Read the model definition and answer for the solid it produces. Units are mm, in the model's axes. Face numbers are marked on the shaded views. A direction names the side the tool comes from. Round coordinates to 2 decimals unless told otherwise and drop trailing zeros. Write each loop counter-clockwise with the first axis right and the second up, starting at its lowest first coordinate (ties: lowest second). Pieces come first, ordered by that corner, then holes. Notation, with made-up numbers: (83, -25) -> (132, -25) arc R34 cw to (132, 9) -> close; hole circle Ø3 at (40, 42). An arc over 180 degrees is marked (long way). Return JSON: item names as keys, results as strings.
from build123d import *

# Parameters (mm, degrees)
SKETCH1_R           = 49.53
BOSS_EXTRUDE1_DEPTH = 15.24
HEX_HOLE_DEPTH      = 13.97
SKETCH5_R           = 4.191
CENTERHOLE_DEPTH    = 72.425504548
SKETCH6_R           = 39.37
CUT_EXTRUDE1_DEPTH  = 11.43
SKETCH7_R           = 3.302
CUT_EXTRUDE2_DEPTH  = 72.684722222
SKETCH8_R           = 49.53
SKETCH8_R_2         = 39.37
CUT_EXTRUDE3_DEPTH  = 11.43
SKETCH9_R           = 49.53
SKETCH9_R_2         = 24.13
SKETCH9_R_3         = 3.302
BOSS_EXTRUDE2_DEPTH = 2.54


with BuildPart() as part:
    # Sketch1 → Boss-Extrude1 (new body)
    with BuildSketch(Plane(origin=(0, 0, 0), x_dir=(1, 0, 0), z_dir=(0, 1, 0))):
        with Locations(Location((0, 0, 0), (0, 0, 90))):
            Circle(SKETCH1_R)
    extrude(amount=BOSS_EXTRUDE1_DEPTH)

    # Sketch4 → Hex hole (cut)
    with BuildSketch(Plane(origin=(0, 15.24, 0), x_dir=(1, 0, 0), z_dir=(0, 1, 0))):
        Polygon((-3.519527241, 6.096), (3.519527241, 6.096), (7.039054482, 0), (3.519527241, -6.096), (-3.519527241, -6.096), (-7.039054482, 0), align=None)
    extrude(amount=-HEX_HOLE_DEPTH, mode=Mode.SUBTRACT)

    # Sketch5 → Centerhole (cut, through all)
    with BuildSketch(Plane(origin=(0, 1.27, 0), x_dir=(1, 0, 0), z_dir=(0, 1, 0))):
        with Locations(Location((0, 0, 0), (0, 0, 270))):
            Circle(SKETCH5_R)
    extrude(amount=-CENTERHOLE_DEPTH, mode=Mode.SUBTRACT)

    # Sketch6 → Cut-Extrude1 (cut)
    with BuildSketch(Plane(origin=(0, 15.24, 0), x_dir=(1, 0, 0), z_dir=(0, 1, 0))):
        with Locations(Location((0, 0, 0), (0, 0, 270))):
            Circle(SKETCH6_R)
        Polygon((12.904933217, 0), (6.452466608, 11.176), (-6.452466608, 11.176), (-12.904933217, 0), (-6.452466608, -11.176), (6.452466608, -11.176), align=None, mode=Mode.SUBTRACT)
    extrude(amount=-CUT_EXTRUDE1_DEPTH, mode=Mode.SUBTRACT)

    # Sketch7 → Cut-Extrude2 (cut, through all)
    with BuildSketch(Plane.XZ):
        with Locations(Location((0, 30.48, 0), (0, 0, 270))):
            Circle(SKETCH7_R)
        with Locations(Location((15.24, 26.396454307, 0), (0, 0, 270))):
            Circle(SKETCH7_R)
        with Locations(Location((26.396454307, 15.24, 0), (0, 0, 270))):
            Circle(SKETCH7_R)
        with Locations(Location((30.48, 0, 0), (0, 0, 270))):
            Circle(SKETCH7_R)
        with Locations(Location((26.396454307, -15.24, 0), (0, 0, 270))):
            Circle(SKETCH7_R)
        with Locations(Location((15.24, -26.396454307, 0), (0, 0, 270))):
            Circle(SKETCH7_R)
        with Locations(Location((0, -30.48, 0), (0, 0, 270))):
            Circle(SKETCH7_R)
        with Locations(Location((-15.24, -26.396454307, 0), (0, 0, 270))):
            Circle(SKETCH7_R)
        with Locations(Location((-26.396454307, -15.24, 0), (0, 0, 270))):
            Circle(SKETCH7_R)
        with Locations(Location((-30.48, 0, 0), (0, 0, 270))):
            Circle(SKETCH7_R)
        with Locations(Location((-26.396454307, 15.24, 0), (0, 0, 270))):
            Circle(SKETCH7_R)
        with Locations(Location((-15.24, 26.396454307, 0), (0, 0, 270))):
            Circle(SKETCH7_R)
    extrude(amount=-CUT_EXTRUDE2_DEPTH, mode=Mode.SUBTRACT)

    # Sketch8 → Cut-Extrude3 (cut)
    with BuildSketch(Plane(origin=(0, 15.24, 0), x_dir=(1, 0, 0), z_dir=(0, 1, 0))):
        with Locations(Location((0, 0, 0), (0, 0, 90))):
            Circle(SKETCH8_R)
        Circle(SKETCH8_R_2, mode=Mode.SUBTRACT)
    extrude(amount=-CUT_EXTRUDE3_DEPTH, mode=Mode.SUBTRACT)

    # Sketch9 → Boss-Extrude2 (add)
    with BuildSketch(Plane(origin=(0, 3.81, 0), x_dir=(1, 0, 0), z_dir=(0, 1, 0))):
        with Locations(Location((0, 0, 0), (0, 0, 90))):
            Circle(SKETCH9_R)
        with Locations(Location((0, 0, 0), (0, 0, 270))):
            Circle(SKETCH9_R_2, mode=Mode.SUBTRACT)
        with Locations(Location((0, 30.48, 0), (0, 0, 90))):
            Circle(SKETCH9_R_3, mode=Mode.SUBTRACT)
        with Locations(Location((15.24, 26.396454307, 0), (0, 0, 90))):
            Circle(SKETCH9_R_3, mode=Mode.SUBTRACT)
        with Locations(Location((26.396454307, 15.24, 0), (0, 0, 90))):
            Circle(SKETCH9_R_3, mode=Mode.SUBTRACT)
        with Locations(Location((30.48, 0, 0), (0, 0, 90))):
            Circle(SKETCH9_R_3, mode=Mode.SUBTRACT)
        with Locations(Location((26.396454307, -15.24, 0), (0, 0, 90))):
            Circle(SKETCH9_R_3, mode=Mode.SUBTRACT)
        with Locations(Location((15.24, -26.396454307, 0), (0, 0, 90))):
            Circle(SKETCH9_R_3, mode=Mode.SUBTRACT)
        with Locations(Location((0, -30.48, 0), (0, 0, 90))):
            Circle(SKETCH9_R_3, mode=Mode.SUBTRACT)
        with Locations(Location((-15.24, -26.396454307, 0), (0, 0, 90))):
            Circle(SKETCH9_R_3, mode=Mode.SUBTRACT)
        with Locations(Location((-26.396454307, -15.24, 0), (0, 0, 90))):
            Circle(SKETCH9_R_3, mode=Mode.SUBTRACT)
        with Locations(Location((-30.48, 0, 0), (0, 0, 90))):
            Circle(SKETCH9_R_3, mode=Mode.SUBTRACT)
        with Locations(Location((-26.396454307, 15.24, 0), (0, 0, 90))):
            Circle(SKETCH9_R_3, mode=Mode.SUBTRACT)
        with Locations(Location((-15.24, 26.396454307, 0), (0, 0, 90))):
            Circle(SKETCH9_R_3, mode=Mode.SUBTRACT)
    extrude(amount=BOSS_EXTRUDE2_DEPTH)


solid = part.part
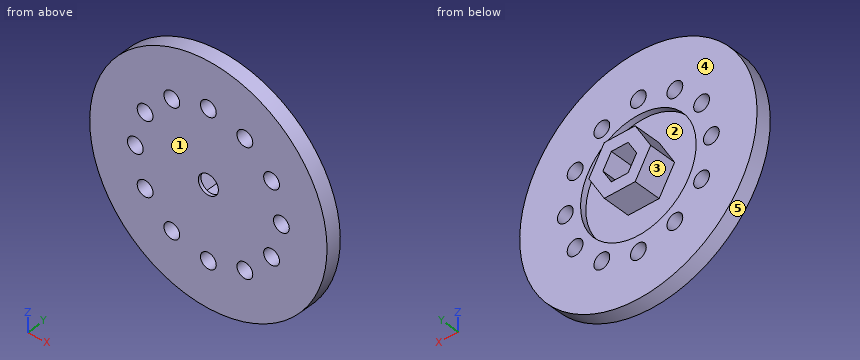
Item 1: Section C-C (z = 15.24) is taken. Give the vertices of the cut face in (x, y), then the cut area to 3 significant figures.
Worked answers:
{"outline": "(-47.13, 0) -> (-29.7, 0) -> (-29.7, 6.35) -> (-47.13, 6.35) -> close; (-23.09, 0) -> (23.09, 0) -> (23.09, 6.35) -> (18.71, 6.35) -> (18.71, 3.81) -> (-18.71, 3.81) -> (-18.71, 6.35) -> (-23.09, 6.35) -> close; (29.7, 0) -> (47.13, 0) -> (47.13, 6.35) -> (29.7, 6.35) -> close", "area": "420 mm2"}
Item 2: Section B-B (x = 0) is taken. Give the vertices of the cut face in (y, z), then the cut area to 3 significant figures.
Worked answers:
{"outline": "(0, -49.53) -> (6.35, -49.53) -> (6.35, -33.78) -> (0, -33.78) -> close; (0, -27.18) -> (6.35, -27.18) -> (6.35, -24.13) -> (3.81, -24.13) -> (3.81, -11.18) -> (15.24, -11.18) -> (15.24, -6.1) -> (1.27, -6.1) -> (1.27, -4.19) -> (0, -4.19) -> close; (0, 4.19) -> (1.27, 4.19) -> (1.27, 6.1) -> (15.24, 6.1) -> (15.24, 11.18) -> (3.81, 11.18) -> (3.81, 24.13) -> (6.35, 24.13) -> (6.35, 27.18) -> (0, 27.18) -> close; (0, 33.78) -> (6.35, 33.78) -> (6.35, 49.53) -> (0, 49.53) -> close", "area": "497 mm2"}
Item 3: For a pull along Z with two mould halves and no side action, classify the marked faces 3, 4 and 5 as released by +Z, released by -Z, zero draft, split by the parting line, or undercut.
Worked answers:
{"face 3": "undercut", "face 4": "zero draft", "face 5": "split by the parting line"}
Item 4: Section A-A (y = 11.5) is taken. Give the vertices of the cut face in (x, z), then the cut area to 3 significant figures.
Worked answers:
{"outline": "(-12.9, 0) -> (-6.45, -11.18) -> (6.45, -11.18) -> (12.9, 0) -> (6.45, 11.18) -> (-6.45, 11.18) -> close; hole (-7.04, 0) -> (-3.52, -6.1) -> (3.52, -6.1) -> (7.04, 0) -> (3.52, 6.1) -> (-3.52, 6.1) -> close", "area": "304 mm2"}
Item 5: Flat-ended cylindrical pins translate along their axes: pin 1 (2 mm diameter, centred on x = 4.5, y = 2.5, fed in from +Z); pin 2 (12 mm diameter, centred on x = -37, z = -2, fed in from +Y); pin 3 (4 mm diameter, centred on x = -4, z = 12.5, fed in from +Y); pin 4 (3.5 mm diameter, centred on x = -1.5, z = 2.5, fed in from +Y). Find the tip coordinate at first contact, or state that the pin passes through.
Worked answers:
{"pin 1": "stops at z = 49.41", "pin 2": "stops at y = 6.35", "pin 3": "stops at y = 15.24", "pin 4": "stops at y = 1.27"}
Item 6: Section D-D (x = -15.24) is taken. Give the vertices of the cut face in (y, z).
Worked answers:
{"outline": "(0, -47.13) -> (6.35, -47.13) -> (6.35, -29.7) -> (0, -29.7) -> close; (0, -23.09) -> (6.35, -23.09) -> (6.35, -18.71) -> (3.81, -18.71) -> (3.81, 18.71) -> (6.35, 18.71) -> (6.35, 23.09) -> (0, 23.09) -> close; (0, 29.7) -> (6.35, 29.7) -> (6.35, 47.13) -> (0, 47.13) -> close"}
Item 7: A tool of negligible diameter and unlimited length cuts with its end or side. For the marked faces 1 and 2, from which of +Z, -Z, +X, -X, +Y, -Y can it reach the whole face along a straight path? Write none if from no direction.
Worked answers:
{"face 1": "+Z, -Z, +X, -X, -Y", "face 2": "+Y"}
Item 8: Straight lines are drawn through the part: L1, parallel to X at y = 2.5, z = 0; L2, parallel to X at y = 5.25, z = -15.24; L3, parallel to X at y = 5.75, z = -27. For each, find the intervals that lie inside material, in ascending order. Write a range as [from, to].
Worked answers:
{"L1": "x = [-49.53, -33.78], [-27.18, -7.04], [7.04, 27.18], [33.78, 49.53]", "L2": "x = [-47.13, -29.7], [-23.09, -18.71], [18.71, 23.09], [29.7, 47.13]", "L3": "x = [-41.52, -18.49], [-11.99, 11.99], [18.49, 41.52]"}
